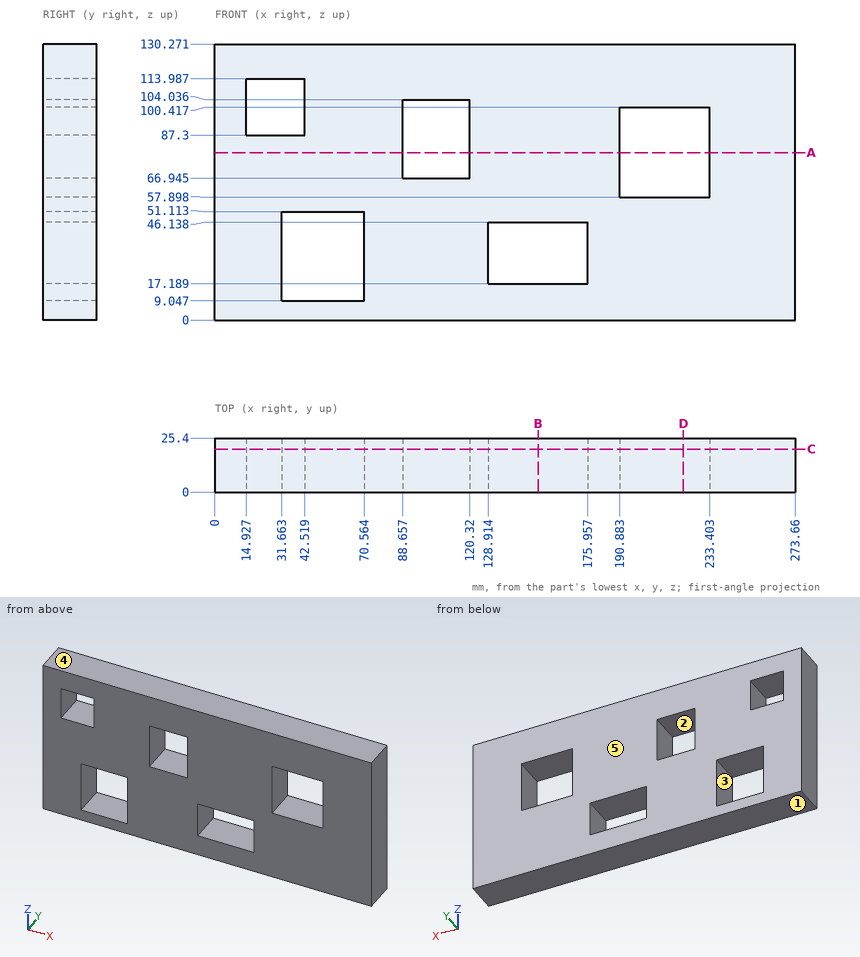
The drawing under review shows one solid part. Ordinate dimensions are in mm from its lowest x, y, z. A direction names the side the tool comes from. Round coordinates to 2 decimals unless told otherwise and drop trailing zeros. Loops run counter-clockwise (first coordinate to the right, second up) from the corner with the lowest first, then second, coordinate; pieces in that order, holes last. Notation, with made-up numbers: (37, -31.75) - (60, -31.75) arc R25 cw to (60, -6.75) - close; hole circle Ø8 at (69.5, 77.25). An arc over 180 degrees is marked (long way). Put each result on its own line as item: value. Start each with the question number.
1. Consider section A-A on z = 79. State the section outline as (x, y) points, plus the area to 3 significant figures.
2. For probe 1 along X at (y, z) = (13.25, 103); probe 2 along X at (y, z) = (3.25, 79.5); probe 3 along Z at (x, y) = (41.5, 10), list the stretches that pass through material, from the lowest coordinate up. Write a range as [from, to].
3. Mouldability with a two-part tool opening along Z and no side actions: class the marked faces 3, 4 and 5 as +Z half, -Z half, draft (parallel to the pull), parting line (faces both ways), or undercut.
4. Consider section D-D on x = 221. State the section outline as (y, z) points.
5. Consider section C-C on y = 20.25. State the section outline as (x, z) points (1 decimal).
6. Consider section B-B on x = 152.5. State the section outline as (y, z) points.
7. For the marked faces 1 and 2, list the 3-axis set-ups (+Z, -Z, +X, -X, +Y, -Y) from which the entire face can be reached by the end or side of a thin tool; tool diameter is ignored.
Result sheet:
1. outline: (0, 0) - (88.66, 0) - (88.66, 25.4) - (0, 25.4) - close; (120.32, 0) - (190.88, 0) - (190.88, 25.4) - (120.32, 25.4) - close; (233.4, 0) - (273.66, 0) - (273.66, 25.4) - (233.4, 25.4) - close
1. area: 5,070 mm^2
2. probe 1: [0, 14.93], [42.52, 88.66], [120.32, 273.66]
2. probe 2: [0, 88.66], [120.32, 190.88], [233.4, 273.66]
2. probe 3: [0, 9.05], [51.11, 87.3], [113.99, 130.27]
3. face 3: undercut
3. face 4: +Z half
3. face 5: draft
4. outline: (0, 0) - (25.4, 0) - (25.4, 57.9) - (0, 57.9) - close; (0, 100.42) - (25.4, 100.42) - (25.4, 130.27) - (0, 130.27) - close
5. outline: (0, 0) - (273.7, 0) - (273.7, 130.3) - (0, 130.3) - close; hole (14.9, 87.3) - (42.5, 87.3) - (42.5, 114) - (14.9, 114) - close; hole (31.7, 9) - (70.6, 9) - (70.6, 51.1) - (31.7, 51.1) - close; hole (88.7, 66.9) - (120.3, 66.9) - (120.3, 104) - (88.7, 104) - close; hole (128.9, 17.2) - (176, 17.2) - (176, 46.1) - (128.9, 46.1) - close; hole (190.9, 57.9) - (233.4, 57.9) - (233.4, 100.4) - (190.9, 100.4) - close
6. outline: (0, 0) - (25.4, 0) - (25.4, 17.19) - (0, 17.19) - close; (0, 46.14) - (25.4, 46.14) - (25.4, 130.27) - (0, 130.27) - close
7. face 1: -Z, +X, -X, +Y, -Y
7. face 2: +Y, -Y
